```python
from build123d import *

# Parameters (mm, degrees)
F0_R     = 47.625
F1_DEPTH = 3.175
F2_R     = 1.58749
F3_D     = 3.175


# Not quite as in the source:
# - a fillet or chamfer is up to 0.001 mm smaller than in the source, because OpenCascade refuses the exact size


with BuildPart() as f1:
    # F0 (on Front) → F1 (new body)
    with BuildSketch(Plane.XZ):
        Circle(F0_R)
    extrude(amount=F1_DEPTH)

    # F2 (radius 1.5875 in the source; OpenCascade refuses exactly that, so slightly less here)
    f2_edges = [f1.edges().sort_by_distance(p)[0] for p in [
        (-47.625, -3.175, 0),
        (-47.625, 0, 0),
    ]]
    fillet(f2_edges, radius=F2_R)

    # F3 (through all)
    with Locations(Plane(origin=(0, 0, 0), x_dir=(1, 0, 0), z_dir=(0, 1, 0))):
        with Locations((0, 0)):
            Hole(F3_D / 2)


solid = f1.part
```
The model under review builds one solid part; all positions refer to its coordinate system, in mm. Round coordinates to 2 decimals unless told otherwise and drop trailing zeros. Order: outer loops, then holes, each group sorted by start corner. A loop starts at its lowest first (then second) coordinate and runs counter-clockwise, first axis right, second up.
(1) Take a section at C-C, the plane y = -0.6. State the section outline as (x, z) points (1 decimal).
Working result:
outline: circle Ø94.6 at (0, 0); hole circle Ø3.2 at (0, 0)
(2) For P1, Ø1.5, axis at x = 34, y = -0.5, coming from the -Z side, flat-tipped, find the tip position at first contact; note if it passes through.
Working result:
P1: stops at z = -33.76
(3) Mouldability with a two-part tool opening along X and no side actions: class faces 1 (the face through (0.34, -1.61, 1.55)), 2 (the face through (-1, -3.175, -10)) as released by +X, released by -X, zero draft, split by the parting line, or undercut.
Working result:
face 1: undercut
face 2: zero draft
(4) Wall thickness on L1, parallel to Z at x = 0, y = -1.4; L2, parallel to Z at x = 0, y = -0.7; L3, parallel to X at y = -0.5, z = 0.5: over which ranges is each line inside the solid? List them lowest first.
Working result:
L1: z = -47.61 to -1.59, 1.59 to 47.61
L2: z = -47.35 to -1.59, 1.59 to 47.35
L3: x = -47.19 to -1.51, 1.51 to 47.19
